The listing builds one solid part. Answer for the finished solid, in the listing's coordinates (mm). Coordinates: 2 decimals unless noted, no trailing zeros. Order: outer loops, then holes, each group sorted by start corner. A loop starts at its lowest first (then second) coordinate and runs counter-clockwise, first axis right, second up. Notation, with made-up numbers: M 83.5,71 L 102.5,71 A9 cw 102.5,76 Z; hole C 25.5,-6 d4. An arc over 180 degrees is marked long. One line per item, written item: value. Start each with the question number.
Q1. Each of these flat-tipped pins is pushed along its axis until it touches: pin 1 Ø3 at (y, z) = (-1, 40) entering from +X; pin 2 Ø1 at (x, z) = (1.5, 34.5) entering from +Y; pin 3 Ø3 at (y, z) = (1.5, 30) entering from -X. Where does it stop, or does it pass through?
Q2. The part is cut by section A-A on y = 0. Give the vertices of the cut face in (x, z).
Q3. The part is cut by section C-C on z = 41. Give the vertices of the cut face in (x, y), then the cut area to 3 significant figures.
Q4. Straight lines are drawn through the part: line 1 along Z through (x, y) = (0.2, 1.55); line 2 along Z through (x, y) = (-0.7, -1.1); line 3 along X through (y, z) = (-0.8, 32.5). For each, find the intervals that lie inside material, in ascending order. Write a range as [from, to].
Q5. Determine the mould class of faces 1 (the cylindrical face through (-0.976, -0.217, 1.246)), 2 (the flat face through (0, 0, 0)), 3 (the cylindrical face through (-0.54, 2.44, 55.99)), 4 (the flat face through (0, 0, 56.5)) for opening direction Z: pulls with the +Z half, pulls with the -Z half, needs draft (parallel to the pull), parting line crosses it, or undercut.
Autodesk Inventor part; units mm, degrees
ref_plane "YZ Plane" through (0, 0, 0) normal (1, 0, 0) x (0, 1, 0)
ref_plane "XZ Plane" through (0, 0, 0) normal (0, 1, 0) x (-1, 0, 0)
ref_plane "XY Plane" through (0, 0, 0) normal (0, 0, 1) x (1, 0, 0)
sketch "Sketch1" plane through (0, 0, 0) normal (0, 0, 1) x (1, 0, 0)
  circle A0 centre (0, 0) radius 1.5
  dimension "d0" = 3
extrude "Extrusion1" add sketch "Sketch1" along normal blind 55.5
sketch "Sketch2" plane through (0, 0, 55.5) normal (0, 0, 1) x (1, 0, 0)
  circle A0 centre (0, 0) radius 1.5
  circle A1 centre (0, 0) radius 2.5
  dimension "d3" = 5
extrude "Extrusion2" add sketch "Sketch2" along normal blind 1 contours A0 | A1
sketch "Sketch3" plane through (0, 0, 0) normal (1, 0, 0) x (0, 1, 0)
  line L0 (-1.5, 55.5) -> (-2.5, 55.5)
  line L1 (-2.5, 55.5) -> (-2.5, 56.5)
  line L2 (-2.5, 56.5) -> (2.5, 56.5)
  line L3 (2.5, 56.5) -> (2.5, 55.5)
  line L4 (2.5, 55.5) -> (1.5, 55.5)
  line L5 (1.5, 55.5) -> (1.5, 0)
  line L6 (1.5, 0) -> (-1.5, 0)
  line L7 (-1.5, 0) -> (-1.5, 55.5)
  line L8 (1.5, 1.5) -> (1, 1.5)
  line L9 (1, 1.5) -> (1, 1)
  line L10 (1, 1) -> (1.5, 1)
  line L11 (1.5, 1) -> (1.5, 1.5)
  line L12 (0, -11.4) -> (0, 68.4)
  point P0 (0, 0)
  dimension "d6" = 54
  dimension "d7" = 0.5
  dimension "d8" = 0.5
revolve "Revolution1" cut sketch "Sketch3" angle 360 about axis through (0, 0, -10) along (0, 0, 1) contours L10 L9 L8 L5
chamfer "Chamfer1" distance 0.5 angle 45 1 edges at (-1.5, 0, 0)
properties part number "Axle" material "Aluminum 6061"
Output:
1. pin 1: stops at x = 1.5
1. pin 2: stops at y = 1.12
1. pin 3: stops at x = -1.5
2. outline: M -2.5,55.5 L -1.5,55.5 L -1.5,1.5 L -1,1.5 L -1,1 L -1.5,1 L -1.5,0.5 L -1,0 L 1,0 L 1.5,0.5 L 1.5,1 L 1,1 L 1,1.5 L 1.5,1.5 L 1.5,55.5 L 2.5,55.5 L 2.5,56.5 L -2.5,56.5 Z
3. outline: C 0,0 d3
3. area: 7.07 mm^2
4. line 1: z = [55.5, 56.5]
4. line 2: z = [0.3, 1], [1.5, 56.5]
4. line 3: x = [-1.27, 1.27]
5. face 1: undercut
5. face 2: pulls with the -Z half
5. face 3: needs draft
5. face 4: pulls with the +Z half
